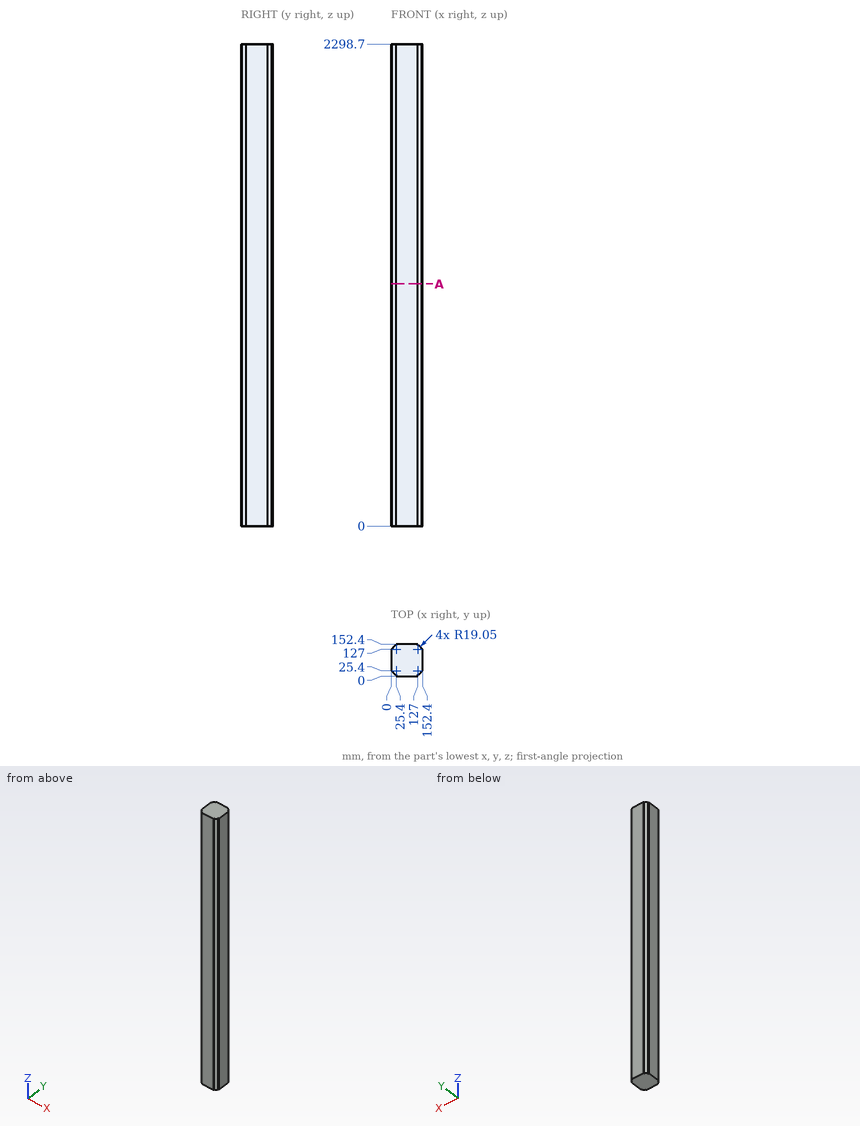
Could you check a few things on this drawing? It's one solid part, dimensions in mm from its lowest x, y, z. Coordinates: 2 decimals unless noted, no trailing zeros. Order: outer loops, then holes, each group sorted by start corner. A loop starts at its lowest first (then second) coordinate and runs counter-clockwise, first axis right, second up. Notation, with made-up numbers: (36, -16.75) -> (95, -16.75) arc R21 cw to (95, 0.25) -> close; hole circle Ø4 at (58, -40). An arc over 180 degrees is marked (long way). Answer in a Markdown table with one row per item.
(1) I want a section at A-A on z = 1155. List the corners of the cut face in (x, y) for me.
Answer key:
| item | result |
|---|---|
| outline | (0, 25.4) -> (6.35, 25.4) arc R19.05 ccw to (25.4, 6.35) -> (25.4, 0) -> (127, 0) -> (127, 6.35) arc R19.05 ccw to (146.05, 25.4) -> (152.4, 25.4) -> (152.4, 127) -> (146.05, 127) arc R19.05 ccw to (127, 146.05) -> (127, 152.4) -> (25.4, 152.4) -> (25.4, 146.05) arc R19.05 ccw to (6.35, 127) -> (0, 127) -> close |
(2) Will these pins go through, and if not, where does the flat tip stop? pin 1 Ø5 at (x, z) = (3.5, 1330) entering from -Y; pin 2 Ø3 at (x, z) = (4, 1450.5) entering from +Y; pin 3 Ø3 at (x, z) = (23, 614) entering from -Y.
Answer key:
| item | result |
|---|---|
| pin 1 | y = 25.4 |
| pin 2 | y = 127 |
| pin 3 | y = 6.37 |
(3) Please list where these lines run through material, in increasing order: probe 1 along X at (y, z) = (127.5, 1176); probe 2 along Y at (x, z) = (128, 1978); probe 3 along Y at (x, z) = (129.5, 1399.5).
Answer key:
| item | result |
|---|---|
| probe 1 | 6.36 to 146.04 |
| probe 2 | 6.38 to 146.02 |
| probe 3 | 6.51 to 145.89 |
